Source: CAD feature listing. Evaluate the final solid. Frame: model axes, mm. Face numbers are marked on the shaded views. Give positions to 0.01 mm unless a question says otherwise; leave off trailing zeros. Write each loop counter-clockwise with the first axis right and the second up, starting at its lowest first coordinate (ties: lowest second). Pieces come first, ordered by that corner, then holes. Notation, with made-up numbers: (-29, -31) - (26, -31) arc R32 cw to (26, 0) - close; hole circle Ø5 at (-34, 54.25). An arc over 180 degrees is marked (long way). One line per question, with ' | ' between items. Start each with the question number.
(1) Pin query (flat end, axial travel): pin 1 (4 mm diameter, centred on x = 11.5, z = -2, fed in from -Y); pin 2 (1 mm diameter, centred on x = 18, y = 2, fed in from +Z). Return the tip coordinate at first contact, or that it passes through.
(2) Draft query along Z for the marked faces 1 and 2. Return one class per face: +Z half, -Z half, draft (parallel to the pull), parting line (faces both ways), or undercut.
(3) Section A-A, the plane x = 6.5. Return loops of the section in (y, z), plus the area to 3 significant figures.
(4) Ray query, line 1 (X direction, y = -1.25, z = 1); line 2 (X direction, y = -1, z = 1.5); line 3 (Y direction, x = 4.5, z = 0). Return the intervals inside material, ascending. Write a range as [from, to].
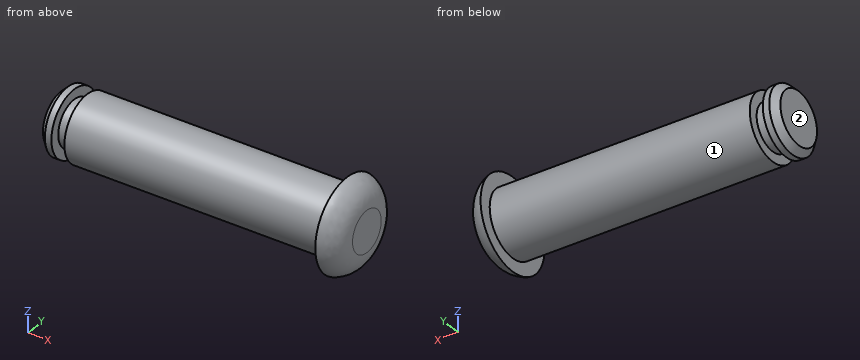
```python
from build123d import *

# Parameters (mm, degrees)
FILLET1_R     = 2
CHAMFER1_SIZE = 0.5


with BuildPart() as part:
    # Sketch1 → Revolve1 (revolve)
    with BuildSketch(Plane.XY):
        Polygon((0, 0), (0, 2.5), (1, 2.5), (1, 1.75), (2, 1.75), (2, 2.5), (22, 2.5), (22, 3.5), (23.5, 3.5), (23.5, 0), align=None)
    revolve(axis=Axis((23.5, 0, 0), (-1, 0, 0)))

    # Fillet1
    # the kernel refuses this fillet: 2 mm, written as the material it takes off along each edge
    with BuildSketch(Plane(origin=(23.5, 0, 0), x_dir=(0, 1, 0), z_dir=(0, 0, 1))) as fillet1_piece_1:
        with BuildLine():
            CenterArc((1.563508327, 2), FILLET1_R, 270, 75.522487814)
            Line((1.563508327, 0), (1.563508327, -0.04))
            Line((1.563508327, -0.04), (3.5, -0.04))
            Line((3.5, -0.04), (3.54, 0))
            ThreePointArc((3.54, 0), (3.54, 0.75), (3.538729833, 1.49))
            Line((3.538729833, 1.49), (3.5, 1.5))
        make_face()
    revolve(axis=Axis((23.5, 0, 0), (-1, 0, 0)), mode=Mode.SUBTRACT)

    # Chamfer1
    chamfer1_edges = [part.edges().sort_by_distance(p)[0] for p in [
        (0, -2.5, 0),
    ]]
    chamfer(chamfer1_edges, length=CHAMFER1_SIZE)


solid = part.part
```
Check sheet entries:
1) pin 1: y = -2.5 | pin 2: z = 2
2) face 1: parting line | face 2: draft
3) outline: circle Ø5 at (0, 0) | area: 19.6 mm²
4) line 1: [0, 23.5] | line 2: [0, 1], [2, 23.49] | line 3: [-2.5, 2.5]
